Autodesk Inventor part; units mm, degrees
ref_plane "YZ Plane" through (0, 0, 0) normal (1, 0, 0) x (0, 1, 0)
ref_plane "XZ Plane" through (0, 0, 0) normal (0, 1, 0) x (-1, 0, 0)
ref_plane "XY Plane" through (0, 0, 0) normal (0, 0, 1) x (1, 0, 0)
sketch "Esquisse1" plane through (0, 0, 0) normal (0, 1, 0) x (-1, 0, 0)
  circle A0 centre (0, 25) radius 4.2
  line L0 (16, 0) -> (-13, 0)
  circle A1 centre (0, -25) radius 4.2
  line L1 (21, 5) -> (-21, 5)
  line L2 (-21, 5) -> (-21, -5)
  line L3 (-21, -5) -> (21, -5)
  line L4 (21, -5) -> (21, 5)
  line L5 (21, 5) -> (-21, -5)
  line L6 (-21, 5) -> (21, -5)
  line L7 (8, 5) -> (-8, 5)
  line L8 (-8, 5) -> (-8, -5)
  line L9 (-8, -5) -> (8, -5)
  line L10 (8, -5) -> (8, 5)
  line L11 (8, 5) -> (-8, -5)
  line L12 (-8, 5) -> (8, -5)
  line L13 (21, 5) -> (21, 35)
  line L14 (-21, 35) -> (-21, 5)
  line L15 (21, 35) -> (-21, 35)
  line L16 (21, -5) -> (21, -35)
  line L17 (-21, -35) -> (-21, -5)
  line L18 (21, -35) -> (-21, -35)
  point P0 (0, 0)
  point P1 (0, 0)
  point P2 (0, 0)
  point P3 (8, -5)
  point P4 (-8, 5)
  dimension "d0" = 8.4
  dimension "d1" = 25
  dimension "d2" = 42
  dimension "d3" = 10
  dimension "d4" = 16
extrude "Extrusion1" add sketch "Esquisse1" along normal blind 10 contours L10 L6 L0 | L0 L5 L10 | L5 L8 L0 | L11 L10 L5 | L11 L8 L5 | L0 L8 L6 | L12 L1 L11 | L12 L3 L11 | L6 L8 L12 | L6 L10 L12 | L1 L14 L15 L13 | L3 L16 L18 L17
sketch "Esquisse2" plane through (0, 10, 0) normal (0, 1, 0) x (1, 0, 0)
  line L0 (-8, -5) -> (-21, -5)
  line L1 (-21, -5) -> (21, -5)
  line L2 (21, -5) -> (21, -14.7)
  line L3 (21, -14.7) -> (-21, -14.7)
  line L4 (-21, -14.7) -> (-21, -5)
  point P0 (0, 0)
  dimension "d8" = 9.7
  dimension "d9" = 42
extrude "Extrusion2" add sketch "Esquisse2" along normal blind 42
sketch "Esquisse3" plane through (0, 10, 0) normal (0, 1, 0) x (1, 0, 0)
  line L0 (21, -14.7) -> (-21, -14.7)
  line L1 (-21, -35) -> (21, -35)
  line L2 (21, -35) -> (21, -14.7)
  line L3 (21, -14.7) -> (-21, -14.7)
  line L4 (-21, -14.7) -> (-21, -35)
  line L5 (21, 35) -> (-21, 35)
  line L6 (-21, 5) -> (21, 5)
  line L7 (21, 5) -> (21, 35)
  line L8 (21, 35) -> (-21, 35)
  line L9 (-21, 35) -> (-21, 5)
  point P0 (0, 0)
  point P1 (-21, -14.7)
extrude "Extrusion3" add sketch "Esquisse3" against normal blind 2
sketch "Esquisse4" plane through (-21, 10, 14.7) normal (0, 0, 1) x (1, 0, 0)
  line L0 (42, 42) -> (0, 42)
  line L1 (42, 0) -> (0, 0)
  line L2 (0, 0) -> (42, 42)
  circle A0 centre (21, 21) radius 13
  line L3 (5.5, 5.5) -> (36.5, 5.5)
  line L4 (36.5, 5.5) -> (36.5, 36.5)
  line L5 (36.5, 36.5) -> (5.5, 36.5)
  line L6 (5.5, 36.5) -> (5.5, 5.5)
  line L7 (5.5, 36.5) -> (36.5, 5.5)
  circle A1 centre (5.5, 36.5) radius 1.75
  circle A2 centre (5.5, 5.5) radius 1.75
  line L8 (21, 36.5) -> (21, 5.5)
  circle A3 centre (36.5, 36.5) radius 1.75
  circle A4 centre (36.5, 5.5) radius 1.75
  point P0 (21, -10)
  point P1 (36.5, 5.5)
  dimension "d14" = 26
  dimension "d20" = 31
  dimension "d21" = 3.5
  dimension "d22" = 3.5
extrude "Extrusion4" cut sketch "Esquisse4" against normal blind 10 contours A2 L6 L2 | L2 L3 A2 | L6 A2 L2 | L2 A2 L3 | A1 L5 L6 | L6 L7 A1 | A0 L7 L2 | L2 L8 A0 | L5 A1 L7 | A4 L7 L3 | L3 L4 A4 | L8 L7 A0 | L8 A0 L2 | L2 A0 L7 | L7 A0 L8 | L7 A4 L4 | A3 L2 L5 | L5 L2 A3 | L2 L4 A3 | L2 A3 L4
fillet "Congé1" radius 5 2 edges at (21, 52, 9.85) (-21, 52, 9.85)
fillet "Congé2" radius 21 4 edges at (21, 5, -35) (-21, 5, -35) (21, 5, 35) (-21, 5, 35)
fillet "Congé3" radius 3 4 edges at (-8, 10, 0) (-8, 0, 0) (8, 0, 0) (8, 10, 0)
properties part number "tete_v2"
Check sheet for the modelled part. Datum: model origin and axes. Units: mm. A direction names the side the tool comes from. Coordinates: 2 decimals unless noted, no trailing zeros. Order: outer loops, then holes, each group sorted by start corner. A loop starts at its lowest first (then second) coordinate and runs counter-clockwise, first axis right, second up. Notation, with made-up numbers: (-1, -37.75) -> (37, -37.75) arc R20 cw to (37, -33.75) -> close; hole circle Ø10 at (44, 9). An arc over 180 degrees is marked (long way). Write item = value, one per line. Start each with the question number.
1) Cross-section at C-C (x = 9). Enter the section's corners in (y, z).
2) Access from +Z, -Z, +X, -X, +Y, -Y to the whole of each face (thin tool, end or side, straight path). Record for faces 1 (the cylindrical face through (0.547, 3.944, -29.164)), 2 (the flat face through (0, 10, 23)), 3 (the cylindrical face through (-7.14, 9.1, -0.07)).
3) Cross-section at D-D (z = 12.5). Enter the section's corners in (x, y).
4) Material ranges on L1, parallel to Y at x = 15.5, z = 7.25; L2, parallel to Z at x = 0, y = 3; L3, parallel to X at y = 46.5, z = 12, recorded low to high.
5) Mould release check, pull along Z, two halves, no side actions. Record for faces 4 (the flat face through (-21, 23, 10)), 5 (the flat face through (0, 8, 25)), 6 (the cylindrical face through (0, 5, -35)), 7 (the flat face through (10, 40, 14.7)): +Z half, -Z half, draft (parallel to the pull), parting line (faces both ways), or undercut.
6) Cross-section at B-B (y = 31). Enter the section's corners in (x, z), then the cut area to 3 significant figures.
7) Cross-section at A-A (y = 15.5). Enter the section's corners in (x, z), then the cut area to 3 significant figures.
8) Go/stop test with flat-tipped pins: P1, Ø1, axis at x = 14, z = -19, coming from the +Y side; P2, Ø2, axis at x = -1.5, y = 16, coming from the -Z side; P3, Ø2, axis at x = 15, y = 14.5, coming from the +Z side. Record where each tip stops, or that it passes through.
Ans:
q1.outline = (0, -32.97) -> (10, -32.97) -> (10, -5) -> (0, -5) -> close; (0, 5) -> (21.62, 5) -> (21.62, 14.7) -> (10, 14.7) -> (10, 32.97) -> (0, 32.97) -> close; (40.38, 5) -> (52, 5) -> (52, 14.7) -> (40.38, 14.7) -> close
q2.face_1 = -Y
q2.face_2 = +Z, +X, -X, +Y
q2.face_3 = -X, +Y
q3.outline = (-21, 0) -> (21, 0) -> (21, 47) arc R5 ccw to (16, 52) -> (-16, 52) arc R5 ccw to (-21, 47) -> close; hole circle Ø3.5 at (-15.5, 15.5); hole circle Ø3.5 at (-15.5, 46.5); hole circle Ø26 at (0, 31); hole circle Ø3.5 at (15.5, 15.5); hole circle Ø3.5 at (15.5, 46.5)
q4.L1 = 0 to 13.75, 17.25 to 44.75, 48.25 to 52
q4.L2 = -35 to -29.2, -20.8 to 20.8, 29.2 to 35
q4.L3 = -21 to -17.25, -13.75 to 13.75, 17.25 to 21
q5.face_4 = draft
q5.face_5 = undercut
q5.face_6 = -Z half
q5.face_7 = +Z half
q6.outline = (-21, 5) -> (-13, 5) -> (-13, 14.7) -> (-20.99, 14.7) arc R21 ccw to (-21, 14) -> close; (13, 5) -> (21, 5) -> (21, 14) arc R21 ccw to (20.99, 14.7) -> (13, 14.7) -> close
q6.area = 155 mm²
q7.outline = (-21, 5) -> (-17.25, 5) -> (-17.25, 14.7) -> (-20.99, 14.7) arc R21 ccw to (-21, 14) -> close; (-13.75, 5) -> (13.75, 5) -> (13.75, 14.7) -> (-13.75, 14.7) -> close; (17.25, 5) -> (21, 5) -> (21, 14) arc R21 ccw to (20.99, 14.7) -> (17.25, 14.7) -> close
q7.area = 339 mm²
q8.P1 = 10
q8.P2 = 5
q8.P3 = 14.7
